```python
from build123d import *

# Parameters (mm, degrees)
F0_W     = 150
F0_H     = 140
F1_DEPTH = 43
F2_R     = 1.5
F3_DEPTH = 25
F4_W     = 34.246223
F4_H     = 17.356102
F5_DEPTH = 5


with BuildPart() as f1:
    # F0 (on Top) → F1 (new body, symmetric)
    with BuildSketch(Plane.XY):
        Rectangle(F0_W, F0_H)
    extrude(amount=F1_DEPTH, both=True)

    # F2 (on face) → F3 (cut)
    with BuildSketch(Plane.XZ.offset(70)):
        with Locations((-69, 37)):
            Circle(F2_R)
        with Locations((69, 37)):
            Circle(F2_R)
        with Locations((45, -37)):
            Circle(F2_R)
        with Locations((-69, -27)):
            Circle(F2_R)
    extrude(amount=-F3_DEPTH, mode=Mode.SUBTRACT)

    # F4 (on face) → F5 (cut)
    with BuildSketch(Plane.XZ.offset(70)):
        with Locations((32.274584, 12.710388)):
            Rectangle(F4_W, F4_H)
    extrude(amount=-F5_DEPTH, mode=Mode.SUBTRACT)


solid = f1.part
```
Check sheet for the modelled part. Datum: model origin and axes. Units: mm. A direction names the side the tool comes from. Give positions to 0.01 mm unless a question says otherwise; leave off trailing zeros. Answer in a Markdown table with one row per item. Add a question column.
Q1. Gauge pin test, flat ends, axial feed: pin 1 Ø5 at (x, z) = (29, 15.5) entering from -Y; pin 2 Ø0.9 at (x, z) = (69.5, 37.5) entering from -Y. Record the tip position at first contact, or that the pin passes through.
Q2. Release check for a two-part mould opening along Z. For faces 1 (the flat face through (-1, 70, 1)), 2 (the flat face through (-1, 1, 43)), 3 (the flat face through (32, -68, 21.388)) record: released by +Z, released by -Z, zero draft, split by the parting line, or undercut.
Q3. Thickness scan on L1, parallel to Z at x = 45, y = -55; L2, parallel to Y at x = 35, z = 8. Record the ranges inside material, lowest first.
Q4. Access from +Z, -Z, +X, -X, +Y, -Y to the whole of each face (thin tool, end or side, straight path). Record for faces 4 (the flat face through (-1, 1, -43)), 5 (the flat face through (32, -65, 13)).
Verdict:
| question | item | result |
|---|---|---|
| 1 | pin 1 | y = -65 |
| 1 | pin 2 | y = -45 |
| 2 | face 1 | zero draft |
| 2 | face 2 | released by +Z |
| 2 | face 3 | undercut |
| 3 | L1 | -43 to -38.5, -35.5 to 43 |
| 3 | L2 | -65 to 70 |
| 4 | face 4 | -Z, +X, -X, +Y, -Y |
| 4 | face 5 | -Y |
